Design review of the part built by this model. Coordinates are the model's own, in mm. A direction names the side the tool comes from. Coordinates: 2 decimals unless noted, no trailing zeros. Loops run counter-clockwise (first coordinate to the right, second up) from the corner with the lowest first, then second, coordinate; pieces in that order, holes last. Notation, with made-up numbers: (37.5, 66) -> (81.5, 66) arc R26 cw to (81.5, 90) -> close; hole circle Ø3 at (9, 26). An arc over 180 degrees is marked (long way). Use one line per item in the form item = value. Start each with the question number.
1. Consider section C-C (z = 13). State the section outline as (x, y) points.
2. Consider section A-A (x = 0). State the section outline as (y, z) points, then the cut area to 3 significant figures.
3. The part is to be moulded in two halves that separate along Y. For faces 1 (the face through (43.986, -44.297, 24.65)), 2 (the face through (-43.986, 44.297, 24.65)), 3 (the face through (23.846, 7.509, 25.35)), say which applies: released by +Y, released by -Y, zero draft, split by the parting line, or undercut.
4. For pin 1 (10 mm diameter, centred on x = -37, z = 41.5, fed in from -Y); pin 2 (1 mm diameter, centred on y = 31, z = 36, fed in from -X); pin 3 (3 mm diameter, centred on y = 35, z = 23, fed in from -X), all flat-tipped, find the tip position at first contact; note any pin that passes through.
5. Machinability: for faces 4 (the face through (0, -50, 25)), 5 (the face through (-40, -30, 38)), which of the approach directions +Z, -Z, +X, -X, +Y, -Y give a long, thin tool a straight path to every point of the face, cutting with its end or side? Answer none if there is none.
6. Wall thickness on line 1 (Y direction, x = 0, z = 28.5); line 2 (Z direction, x = -40, y = -35.5); line 3 (Y direction, x = 4, z = 29): over which ranges is each line inside the solid? List them lowest first. Write a range as from..to.
7. Consider section B-B (y = 20). State the section outline as (x, z) points, then the cut area to 3 significant figures.
from build123d import *

# Parameters (mm, degrees)
F1_DEPTH = 50
F2_R     = 25
F3_DEPTH = 50.001
F4_W     = 20
F4_H     = 20
F5_DEPTH = 25


with BuildPart() as f1:
    # F0 (on Top) → F1 (new body)
    with BuildSketch(Plane.XY):
        with BuildLine():
            ThreePointArc((50, 30), (44.142136, 44.142136), (30, 50))
            Line((30, 50), (-30, 50))
            ThreePointArc((-30, 50), (-44.142136, 44.142136), (-50, 30))
            Line((-50, 30), (-50, -30))
            ThreePointArc((-50, -30), (-44.142136, -44.142136), (-30, -50))
            Line((-30, -50), (30, -50))
            ThreePointArc((30, -50), (44.142136, -44.142136), (50, -30))
            Line((50, -30), (50, 30))
        make_face()
    extrude(amount=F1_DEPTH)

    # F2 (on face) → F3 (cut, through all)
    with BuildSketch(Plane.XY.offset(50)):
        Circle(F2_R)
    extrude(amount=-F3_DEPTH, mode=Mode.SUBTRACT)

    # F4 (on face) → F5 (cut)
    with BuildSketch(Plane.XY.offset(50)):
        with Locations((-40, -40)):
            Rectangle(F4_W, F4_H)
    extrude(amount=-F5_DEPTH, mode=Mode.SUBTRACT)


solid = f1.part
Geometry check:
q1.outline = (-50, -30) arc R20 ccw to (-30, -50) -> (30, -50) arc R20 ccw to (50, -30) -> (50, 30) arc R20 ccw to (30, 50) -> (-30, 50) arc R20 ccw to (-50, 30) -> close; hole circle Ø50 at (0, 0)
q2.outline = (-50, 0) -> (-25, 0) -> (-25, 50) -> (-50, 50) -> close; (25, 0) -> (50, 0) -> (50, 50) -> (25, 50) -> close
q2.area = 2,500 mm²
q3.face_1 = released by -Y
q3.face_2 = released by +Y
q3.face_3 = undercut
q4.pin_1 = -30
q4.pin_2 = -49.99
q4.pin_3 = -49.69
q5.face_4 = +Z, -Z, +X, -X, -Y
q5.face_5 = +Z, -X, -Y
q6.line_1 = -50..-25, 25..50
q6.line_2 = 0..25
q6.line_3 = -50..-24.68, 24.68..50
q7.outline = (-50, 0) -> (-15, 0) -> (-15, 50) -> (-50, 50) -> close; (15, 0) -> (50, 0) -> (50, 50) -> (15, 50) -> close
q7.area = 3,500 mm²
